The listing builds one solid part. Answer for the finished solid, in the listing's coordinates (mm). Coordinates: 2 decimals unless noted, no trailing zeros. Order: outer loops, then holes, each group sorted by start corner. A loop starts at its lowest first (then second) coordinate and runs counter-clockwise, first axis right, second up. Notation, with made-up numbers: (-12, -0.75) -> (28, -0.75) arc R27 cw to (28, 16.25) -> close; hole circle Ø2 at (10.25, 27.5). An arc over 180 degrees is marked (long way). Put each result on its own line as item: value. Start each with the question number.
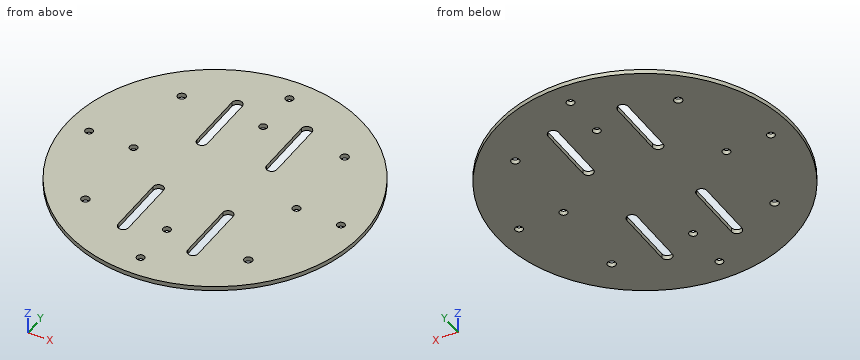
```python
from build123d import *

# Parameters (mm, degrees)
IZIM1_R                              = 100
Y_KSEKLIK_EKSTR_ZYON1_DEPTH          = 30
M5_HELISARMAL_I_IN_Z_VANA_MATKAB_1_D = 5.2
KES_EKSTR_ZYON1_DEPTH                = 145.568322948
M5_BO_LUKLU_DELIK2_D                 = 5.5
IZIM20_R                             = 183.537558205
KES_EKSTR_ZYON2_DEPTH                = 27


with BuildPart() as part:
    # Çizim1 → Yükseklik-Ekstrüzyon1 (new body)
    with BuildSketch(Plane.XY):
        Circle(IZIM1_R)
    extrude(amount=Y_KSEKLIK_EKSTR_ZYON1_DEPTH)

    # M5 Helisarmal için Zıvana matkabı1 (through all)
    with Locations(Plane.XY.offset(30)):
        with Locations((-85, 0), (-55, 0), (0, 55), (0, 85), (55, 0), (85, 0), (0, -55), (0, -85)):
            Hole(M5_HELISARMAL_I_IN_Z_VANA_MATKAB_1_D / 2)

    # Çizim9 → Kes-Ekstrüzyon1 (cut, through all)
    with BuildSketch(Plane.XY.offset(30)):
        with BuildLine():
            Line((27, 65), (27, 25))
            ThreePointArc((27, 25), (23.5, 21.5), (20, 25))
            Line((20, 25), (20, 65))
            ThreePointArc((20, 65), (23.5, 68.5), (27, 65))
        make_face()
        with BuildLine():
            Line((-20, 65), (-20, 25))
            ThreePointArc((-20, 25), (-23.5, 21.5), (-27, 25))
            Line((-27, 25), (-27, 65))
            ThreePointArc((-27, 65), (-23.5, 68.5), (-20, 65))
        make_face()
        with BuildLine():
            Line((-20, -25), (-20, -65))
            ThreePointArc((-20, -65), (-23.5, -68.5), (-27, -65))
            Line((-27, -65), (-27, -25))
            ThreePointArc((-27, -25), (-23.5, -21.5), (-20, -25))
        make_face()
        with BuildLine():
            Line((20, -65), (20, -25))
            ThreePointArc((20, -25), (23.5, -21.5), (27, -25))
            Line((27, -25), (27, -65))
            ThreePointArc((27, -65), (23.5, -68.5), (20, -65))
        make_face()
    extrude(amount=-KES_EKSTR_ZYON1_DEPTH, mode=Mode.SUBTRACT)

    # M5 Boşluklu Delik2 (through all)
    with Locations(Plane.XY.offset(30)):
        with Locations((-55, 55), (55, 55), (55, -55), (-55, -55)):
            Hole(M5_BO_LUKLU_DELIK2_D / 2)

    # Çizim20 → Kes-Ekstrüzyon2 (cut)
    with BuildSketch(Plane.XY.offset(30)):
        with Locations((0, 8.479468632)):
            Circle(IZIM20_R)
    extrude(amount=-KES_EKSTR_ZYON2_DEPTH, mode=Mode.SUBTRACT)


solid = part.part
```
(1) The part is cut by section D-D on y = -27.5. Determine the outline of the cut face in (x, z).
(2) Each of these flat-tipped pins is pushed along its axis until it touches: P1, Ø4.5, axis at x = 0, y = 55, coming from the +Z side; P2, Ø0.9, axis at y = 52, z = 1.5, coming from the +X side; P3, Ø1.5, axis at x = -13, z = 2, coming from the +Y side; P4, Ø0.9, axis at y = -40.5, z = 1.5, coming from the +X side. Where does it stop, or does it pass through?
(3) The part is cut by section A-A on z = 0.85. Count the separate pieces of the cut face and the enclosed holes in it, plus the area to 3 significant figures.
(4) The part is cut by section C-C on x = -23.5. Determine the outline of the cut face in (y, z).
(5) The part is cut by section B-B on y = 0. Determine the outline of the cut face in (x, z), plus the area to 3 significant figures.
(6) Find the intervals of material crossed by L1, parallel to Y at x = 0, z = 1.75; L2, parallel to Y at x = 55, z = 1.8; L3, parallel to X at y = -46, z = 0.9, in increasing order.
Worked out:
1. outline: (-96.14, 0) -> (-27, 0) -> (-27, 3) -> (-96.14, 3) -> close; (-20, 0) -> (20, 0) -> (20, 3) -> (-20, 3) -> close; (27, 0) -> (96.14, 0) -> (96.14, 3) -> (27, 3) -> close
2. P1: through
2. P2: x = 85.69
2. P3: y = 99.25
2. P4: x = 91.63
3. separate pieces: 1
3. enclosed holes: 16
3. area: 29,900 mm2
4. outline: (-97.2, 0) -> (-68.5, 0) -> (-68.5, 3) -> (-97.2, 3) -> close; (-21.5, 0) -> (21.5, 0) -> (21.5, 3) -> (-21.5, 3) -> close; (68.5, 0) -> (97.2, 0) -> (97.2, 3) -> (68.5, 3) -> close
5. outline: (-100, 0) -> (-87.6, 0) -> (-87.6, 3) -> (-100, 3) -> close; (-82.4, 0) -> (-57.6, 0) -> (-57.6, 3) -> (-82.4, 3) -> close; (-52.4, 0) -> (52.4, 0) -> (52.4, 3) -> (-52.4, 3) -> close; (57.6, 0) -> (82.4, 0) -> (82.4, 3) -> (57.6, 3) -> close; (87.6, 0) -> (100, 0) -> (100, 3) -> (87.6, 3) -> close
5. area: 538 mm2
6. L1: -100 to -87.6, -82.4 to -57.6, -52.4 to 52.4, 57.6 to 82.4, 87.6 to 100
6. L2: -83.52 to -57.75, -52.25 to -2.6, 2.6 to 52.25, 57.75 to 83.52
6. L3: -88.79 to -27, -20 to 20, 27 to 88.79
